For this review, take the finished solid that the model builds, in its own axes (mm). Face numbers are marked on the shaded views. A direction names the side the tool comes from. Coordinates: 2 decimals unless noted, no trailing zeros. Write each loop counter-clockwise with the first axis right and the second up, starting at its lowest first coordinate (ties: lowest second). Pieces come first, ordered by that corner, then holes. Notation, with made-up numbers: (-26.5, 88.5) -> (6.5, 88.5) arc R18 ccw to (6.5, 107.5) -> close; hole circle Ø7 at (-13.75, -3). An arc over 180 degrees is marked (long way). One line per item, written item: value. Start each with the question number.
1) For probe 1 along Y at (x, z) = (63.5, 49); probe 2 along Z at (x, y) = (3, 50.5); probe 3 along Z at (x, y) = (27, 46), list the stretches that pass through material, from the lowest coordinate up. Write a range as from..to.
2) Add section A-A (y = 55). State how many separate pieces and enclosed holes the cut face has, and give its area (3 significant figures).
3) Machinability: for the marked faces 1, 2 and 3, which of the approach directions +Z, -Z, +X, -X, +Y, -Y give a long, thin tool a straight path to every point of the face, cutting with its end or side? Answer none if there is none.
4) Mouldability with a two-part tool opening along X and no side actions: class the marked faces 4, 5 and 6 as released by +X, released by -X, zero draft, split by the parting line, or undercut.
5) For pin 1 Ø14.5 at (x, z) = (-57.65, 56.41) entering from +Y; pin 2 Ø10 at (y, z) = (44.5, -27.5) entering from +X; pin 3 Ø4 at (x, y) = (-10.5, -33) entering from -Z, all flat-tipped, find the tip position at first contact; note any pin that passes through.
6) Add section C-C (y = -33.5). State the section outline as (x, z) points, and give its area (3 significant figures).
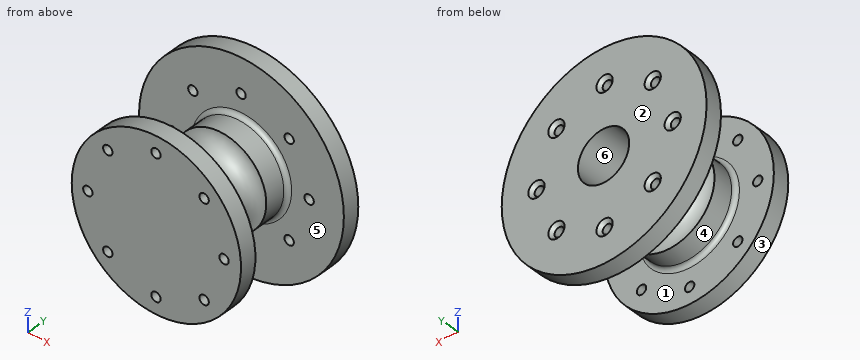
from build123d import *

# Parameters (mm, degrees)
CSK_FOR_M10_CROSS_COUNTERSUNK_HEAD_SCREW_D           = 11
CSK_FOR_M10_CROSS_COUNTERSUNK_HEAD_SCREW_CSINK_D     = 19
CSK_FOR_M10_CROSS_COUNTERSUNK_HEAD_SCREW_CSINK_ANGLE = 92
CIRPATTERN1_COUNT                                    = 8
SKETCH4_R                                            = 30
CUT_EXTRUDE1_DEPTH                                   = 88


with BuildPart() as part:
    # Sketch1 → Revolve1 (revolve)
    with BuildSketch(Plane.XY, mode=Mode.PRIVATE) as revolve1_sk:
        with BuildLine():
            Line((-0.742985442, 69.00355741), (119.257014558, 69.00355741))
            Line((119.257014558, 69.00355741), (119.257014558, 49.00355741))
            Line((119.257014558, 49.00355741), (58.145903447, 49.00355741))
            ThreePointArc((58.145903447, 49.00355741), (54.610369541, 47.539091316), (53.145903447, 44.00355741))
            Line((53.145903447, 44.00355741), (53.145903447, 19.678538808))
            ThreePointArc((53.145903447, 19.678538808), (33.145903447, -0.321461192), (53.145903447, -20.321461192))
            Line((53.145903447, -20.321461192), (53.145903447, -44.00355741))
            ThreePointArc((53.145903447, -44.00355741), (54.610369541, -47.539091316), (58.145903447, -49.00355741))
            Line((58.145903447, -49.00355741), (98.423681225, -49.00355741))
            Line((98.423681225, -49.00355741), (98.423681225, -69.00355741))
            Line((98.423681225, -69.00355741), (-0.742985442, -69.00355741))
            Line((-0.742985442, -69.00355741), (-0.742985442, -7.70421595))
            ThreePointArc((-0.742985442, -7.70421595), (7.739959352, 0), (-0.742985442, 7.70421595))
            Line((-0.742985442, 7.70421595), (-0.742985442, 69.00355741))
        make_face()
    revolve(revolve1_sk.sketch.rotate(Axis((-0.742985442, 69.00355741, 0), (0, -1, 0)), 180), axis=Axis((-0.742985442, 69.00355741, 0), (0, -1, 0)))

    # CSK for M10 Cross Countersunk Head Screw1 (through all)
    with Locations(Plane(origin=(0, 69.00355741, 0), x_dir=(1, 0, 0), z_dir=(0, 1, 0))):
        with Locations((78.534069327, 0)):
            csk_for_m10_cross_countersunk_head_screw = CounterSinkHole(CSK_FOR_M10_CROSS_COUNTERSUNK_HEAD_SCREW_D / 2, CSK_FOR_M10_CROSS_COUNTERSUNK_HEAD_SCREW_CSINK_D / 2, counter_sink_angle=CSK_FOR_M10_CROSS_COUNTERSUNK_HEAD_SCREW_CSINK_ANGLE)

    # CirPattern1: CSK for M10 Cross Countersunk Head Screw1 ×8 about axis
    cirpattern1_axis = Axis((-1.242977, 0, 0), (0, 1, 0))
    for i in range(1, CIRPATTERN1_COUNT):
        add(csk_for_m10_cross_countersunk_head_screw.rotate(cirpattern1_axis, i * 360 / CIRPATTERN1_COUNT), mode=Mode.SUBTRACT)

    # Sketch4 → Cut-Extrude1 (cut)
    with BuildSketch(Plane(origin=(0, 69.00355741, 0), x_dir=(1, 0, 0), z_dir=(0, 1, 0))):
        with Locations(Location((0, 0, 0), (0, 0, 270))):
            Circle(SKETCH4_R)
    extrude(amount=-CUT_EXTRUDE1_DEPTH, mode=Mode.SUBTRACT)


solid = part.part
Numbers:
1. probe 1: -69..-49, 49..69
1. probe 2: -119.94..-83.28, -76.28..-29.85, 29.85..76.28, 83.28..119.94
1. probe 3: -46.68..-13.08, 13.08..46.68
2. separate pieces: 1
2. enclosed holes: 9
2. area: 41,700 mm²
3. face 1: none
3. face 2: +Z, -Z, +X, -X, +Y
3. face 3: -Y
4. face 4: split by the parting line
4. face 5: zero draft
4. face 6: undercut
5. pin 1: y = 66.83
5. pin 2: x = 116.55
5. pin 3: z = -53.33
6. outline: circle Ø107.78 at (-0.74, 0)
6. area: 9,120 mm²
